Part model, mm, in its own coordinate system. A direction names the side the tool comes from. Round coordinates to 2 decimals unless told otherwise and drop trailing zeros. Write each loop counter-clockwise with the first axis right and the second up, starting at its lowest first coordinate (ties: lowest second). Pieces come first, ordered by that corner, then holes. Notation, with made-up numbers: (-33, 46.25) -> (21, 46.25) arc R22 cw to (21, 73.25) -> close; hole circle Ø2 at (-12.5, -19.5). An arc over 180 degrees is marked (long way). Return JSON: item names as keys, results as strings. Group by question number.
(1) Drop flat-ended pins along their axis: pin 1 Ø1.6 at (y, z) = (-2, 3) entering from -X; pin 2 Ø2.5 at (x, y) = (1.5, -2) entering from +Z; pin 3 Ø1.3 at (x, z) = (0.5, 4.5) entering from +Y. Give the stop position or say it passes through.
(2) Saw through at A-A (z = -21). List the corners of the cut face in (x, y).
(3) Drill centre lines: L1, parallel to X at y = -6.25, z = 1.5; L2, parallel to X at y = -5.25, z = -23; L3, parallel to Y at x = -1.35, z = -6.35 (3 decimals). Where is each one in solid material? Low to high. Write a range as from..to.
(4) Mould opens along X. For faces 4 (the flat face through (-4.324, -2.161, -4.626)), 5 (the cylindrical face through (-8.45, -6.13, 2.94)), 6 (the cylindrical face through (3.684, -3.131, -25.099)) say: +X half, -X half, draft (parallel to the pull), parting line (faces both ways), or undercut.
(5) Tool access for faces 1 (the flat face through (-14, -2, 3)), 2 (the flat face through (-3, -6.35, -13)), 3 (the flat face through (7.8, -13.4, 4.19)): list every direction of +Z, -Z, +X, -X, +Y, -Y with a clear straight run to the whole face (end or side of a thin tool).
(6) Saw through at C-C (z = -6.35). List the corners of the cut face in (x, y) (3 decimals), plus the area to 3 significant figures.
(7) Saw through at B-B (y = -8.25). List the corners of the cut face in (x, z) (3 decimals), plus the area to 3 significant figures.
(8) Saw through at D-D (x = -12.5). List the corners of the cut face in (y, z).
from build123d import *

# Parameters (mm, degrees)
SKETCH1_R                     = 19.05
SKETCH1_R_2                   = 0.5
BOSS_EXTRUDE1_DEPTH           = 6.35
M3_CLEARANCE_HOLE1_D          = 3.2
M3_CLEARANCE_HOLE1_DEPTH      = 29.72
M3_CLEARANCE_HOLE1_TIP        = 0.96137699
SKETCH4_W                     = 37.608509676
SKETCH4_H                     = 0.25
CUT_EXTRUDE1_DEPTH            = 28.679008291
CBORE_FOR_M2_SHCS1_AT_2_COUNT = 2
CBORE_FOR_M2_SHCS1_AT_2_PITCH = 19.05
CUT_EXTRUDE2_DEPTH            = 10
FILLET1_R                     = 2.38125
SKETCH12_W                    = 55.779861043
SKETCH12_H                    = 27.835929003
CUT_EXTRUDE3_DEPTH            = 28.679008452
SKETCH13_W                    = 3
SKETCH13_H                    = 3
BOSS_EXTRUDE2_DEPTH           = 2.5
FILLET2_R                     = 0.5
SKETCH14_W                    = 1.5875
SKETCH14_H                    = 1.4625
CUT_EXTRUDE4_DEPTH            = 28.481584743
SKETCH15_W                    = 3.175
SKETCH15_H                    = 6.35
SKETCH15_W_2                  = 4.7625
BOSS_EXTRUDE3_DEPTH           = 25.4
M2_CLEARANCE_HOLE1_D          = 2.2
M2_CLEARANCE_HOLE1_DEPTH      = 28.35
M2_CLEARANCE_HOLE1_TIP        = 0.660946681
CUT_EXTRUDE5_DEPTH            = 2.5
FILLET3_R                     = 1
FILLET4_R                     = 1


with BuildPart() as part:
    # Sketch1 → Boss-Extrude1 (new body)
    with BuildSketch(Plane.XY):
        Circle(SKETCH1_R)
        with Locations((-12.7, 0)):
            Circle(SKETCH1_R_2, mode=Mode.SUBTRACT)
        with Locations((12.7, 0)):
            Circle(SKETCH1_R_2, mode=Mode.SUBTRACT)
        Circle(SKETCH1_R_2, mode=Mode.SUBTRACT)
    extrude(amount=BOSS_EXTRUDE1_DEPTH)

    # M3 Clearance Hole1
    with Locations(Plane(origin=(-15.665967818, 20.219646462, 6.35), x_dir=(1, 0, 0), z_dir=(0, 0, 1))):
        with Locations((15.665967818, -5.554949625), (2.965967818, -27.551994881), (28.365967818, -27.551994881)):
            Hole(M3_CLEARANCE_HOLE1_D / 2, depth=M3_CLEARANCE_HOLE1_DEPTH)
            with Locations((0, 0, -(M3_CLEARANCE_HOLE1_DEPTH + M3_CLEARANCE_HOLE1_TIP / 2))):  # 118° drill point
                Cone(0, M3_CLEARANCE_HOLE1_D / 2, M3_CLEARANCE_HOLE1_TIP, mode=Mode.SUBTRACT)

    # Sketch4 → Cut-Extrude1 (cut, through all)
    with BuildSketch(Plane(origin=(0, 0, 0), x_dir=(-1, 0, 0), z_dir=(0, 0, -1))):
        with Locations((0, -3.175)):
            Rectangle(SKETCH4_W, SKETCH4_H)
    extrude(amount=-CUT_EXTRUDE1_DEPTH, mode=Mode.SUBTRACT)


with BuildPart() as cut_extrude1_piece_1:
    # of the separate pieces the step leaves, piece 1, a body of its own (cut_extrude1_pieces)
    add(part.part.solids().sort_by_distance((18.804254838, -3.05, 0))[0])


with BuildPart() as cut_extrude1_piece_2:
    # of the separate pieces the step leaves, piece 2, a body of its own (cut_extrude1_pieces)
    add(part.part.solids().sort_by_distance((-18.761996162, -3.3, 0))[0])


with BuildPart() as cbore_for_m2_shcs1_tool:
    # Sketch9 → CBORE for M2 SHCS1 (revolve)
    with BuildSketch(Plane(origin=(-9.525, 19.05, 3.175), x_dir=(0, 0, 1), z_dir=(1, 0, 0))):
        Polygon((0, 0), (0, 38.1), (1.1, 38.1), (1.1, 2), (2.2, 2), (2.2, 0), align=None)
    cbore_for_m2_shcs1 = revolve(axis=Axis((-9.525, 25.4, 3.175), (0, -1, 0)))


with BuildPart() as cut_extrude1_piece_1_1:
    add(cut_extrude1_piece_1.part)

    # CBORE for M2 SHCS1: cut by cbore_for_m2_shcs1_tool
    add(cbore_for_m2_shcs1_tool.part, mode=Mode.SUBTRACT)


with BuildPart() as cut_extrude1_piece_2_1:
    add(cut_extrude1_piece_2.part)

    # CBORE for M2 SHCS1: cut by cbore_for_m2_shcs1_tool
    add(cbore_for_m2_shcs1_tool.part, mode=Mode.SUBTRACT)


with BuildPart() as cbore_for_m2_shcs1_at_2_tool:
    # CBORE for M2 SHCS1 at 2: CBORE for M2 SHCS1 ×2
    with Locations(*[(i * CBORE_FOR_M2_SHCS1_AT_2_PITCH, 0, 0) for i in range(1, CBORE_FOR_M2_SHCS1_AT_2_COUNT)]):
        add(cbore_for_m2_shcs1)


with BuildPart() as cut_extrude1_piece_1_2:
    add(cut_extrude1_piece_1_1.part)

    # CBORE for M2 SHCS1 at 2: cut by cbore_for_m2_shcs1_at_2_tool
    add(cbore_for_m2_shcs1_at_2_tool.part, mode=Mode.SUBTRACT)

    # Fillet1
    fillet1_edges = [cut_extrude1_piece_1_2.edges().sort_by_distance(p)[0] for p in [
        (-0.5, 0, 0),
        (-13.2, 0, 0),
        (12.2, 0, 0),
        (-13.2, 0, 6.35),
        (12.2, 0, 6.35),
        (-0.5, 0, 6.35),
    ]]
    fillet(fillet1_edges, radius=FILLET1_R)

    # Sketch12 → Cut-Extrude3 (cut, through all)
    with BuildSketch(Plane.XY):
        with Locations((0.042756797, 10.867964502)):
            Rectangle(SKETCH12_W, SKETCH12_H)
    extrude(amount=CUT_EXTRUDE3_DEPTH, mode=Mode.SUBTRACT)


with BuildPart() as cut_extrude1_piece_2_2:
    add(cut_extrude1_piece_2_1.part)

    # CBORE for M2 SHCS1 at 2: cut by cbore_for_m2_shcs1_at_2_tool
    add(cbore_for_m2_shcs1_at_2_tool.part, mode=Mode.SUBTRACT)

    # Sketch11 → Cut-Extrude2 (cut)
    with BuildSketch(Plane.XZ.offset(19.05)):
        Polygon((-10.679700538, 5.175), (-11.834401077, 3.175), (-10.679700538, 1.175), (-8.370299462, 1.175), (-7.215598923, 3.175), (-8.370299462, 5.175), align=None)
        Polygon((8.370299462, 5.175), (7.215598923, 3.175), (8.370299462, 1.175), (10.679700538, 1.175), (11.834401077, 3.175), (10.679700538, 5.175), align=None)
    extrude(amount=-CUT_EXTRUDE2_DEPTH, mode=Mode.SUBTRACT)

    # Sketch13 → Boss-Extrude2 (add)
    with BuildSketch(Plane(origin=(0, -3.3, 0), x_dir=(1, 0, 0), z_dir=(0, 1, 0))):
        with Locations((-15.5, -3.175)):
            Rectangle(SKETCH13_W, SKETCH13_H)
        with Locations((15.5, -3.175)):
            Rectangle(SKETCH13_W, SKETCH13_H)
    extrude(amount=BOSS_EXTRUDE2_DEPTH)

    # Fillet2
    fillet2_edges = [cut_extrude1_piece_2_2.edges().sort_by_distance(p)[0] for p in [
        (17, -3.3, 3.175),
        (17, -2.05, 4.675),
        (15.5, -3.3, 1.675),
        (17, -2.05, 1.675),
        (14, -3.3, 3.175),
        (14, -2.05, 1.675),
        (15.5, -3.3, 4.675),
        (14, -2.05, 4.675),
        (17, -0.8, 3.175),
        (15.5, -0.8, 1.675),
        (14, -0.8, 3.175),
        (15.5, -0.8, 4.675),
        (-15.5, -3.3, 1.675),
        (-14, -2.05, 1.675),
        (-17, -3.3, 3.175),
        (-17, -2.05, 1.675),
        (-15.5, -3.3, 4.675),
        (-17, -2.05, 4.675),
        (-14, -3.3, 3.175),
        (-14, -2.05, 4.675),
        (-15.5, -0.8, 1.675),
        (-17, -0.8, 3.175),
        (-15.5, -0.8, 4.675),
        (-14, -0.8, 3.175),
    ]]
    fillet(fillet2_edges, radius=FILLET2_R)

    # Sketch14 → Cut-Extrude4 (cut, through all)
    with BuildSketch(Plane(origin=(0, 0, 0), x_dir=(-1, 0, 0), z_dir=(0, 0, -1))):
        with Locations((0, -4.03125)):
            Rectangle(SKETCH14_W, SKETCH14_H)
    extrude(amount=-CUT_EXTRUDE4_DEPTH, mode=Mode.SUBTRACT)

    # Sketch15 → Boss-Extrude3 (add)
    with BuildSketch(Plane(origin=(0, 0, 0), x_dir=(-1, 0, 0), z_dir=(0, 0, -1))):
        with Locations((-2.38125, -3.175)):
            Rectangle(SKETCH15_W, SKETCH15_H)
        with Locations((3.175, -3.175)):
            Rectangle(SKETCH15_W_2, SKETCH15_H)
    extrude(amount=BOSS_EXTRUDE3_DEPTH)

    # M2 Clearance Hole1
    with Locations(Plane.ZY.offset(5.55625)):
        with Locations((-6.35, -3.175)):
            Hole(M2_CLEARANCE_HOLE1_D / 2, depth=M2_CLEARANCE_HOLE1_DEPTH)
            with Locations((0, 0, -(M2_CLEARANCE_HOLE1_DEPTH + M2_CLEARANCE_HOLE1_TIP / 2))):  # 118° drill point
                Cone(0, M2_CLEARANCE_HOLE1_D / 2, M2_CLEARANCE_HOLE1_TIP, mode=Mode.SUBTRACT)

    # Sketch18 → Cut-Extrude5 (cut)
    with BuildSketch(Plane.ZY.offset(5.55625)):
        Polygon((-7.504700538, -1.175), (-5.195299462, -1.175), (-4.040598923, -3.175), (-5.195299462, -5.175), (-7.504700538, -5.175), (-8.659401077, -3.175), align=None)
    extrude(amount=-CUT_EXTRUDE5_DEPTH, mode=Mode.SUBTRACT)

    # Fillet3
    fillet3_edges = [cut_extrude1_piece_2_2.edges().sort_by_distance(p)[0] for p in [
        (3.96875, -4.825, 0),
        (2.38125, -6.35, 0),
        (0.79375, -3.175, -25.4),
        (2.38125, 0, -25.4),
        (3.96875, -3.175, -25.4),
        (2.38125, -6.35, -25.4),
        (-3.175, -6.35, 0),
        (-5.55625, -4.825, 0),
        (-0.79375, -3.175, -25.4),
        (-3.175, -6.35, -25.4),
        (-5.55625, -3.175, -25.4),
        (-3.175, 0, -25.4),
    ]]
    fillet(fillet3_edges, radius=FILLET3_R)

    # Fillet4
    fillet4_edges = [cut_extrude1_piece_2_2.edges().sort_by_distance(p)[0] for p in [
        (2.38125, 0, 0),
        (-3.175, 0, 0),
    ]]
    fillet(fillet4_edges, radius=FILLET4_R)


solid = cut_extrude1_piece_2_2.part
Computed values:
{
 "1": {"pin 1": "x = -17", "pin 2": "z = 0", "pin 3": "y = -3.3"},
 "2": {"outline": "(-5.56, -6.35) -> (-0.79, -6.35) -> (-0.79, 0) -> (-5.56, 0) -> close; (0.79, -6.35) -> (3.97, -6.35) -> (3.97, 0) -> (0.79, 0) -> close"},
 "3": {"L1": "-18..-13.88, -11.52..11.52, 13.88..18", "L2": "-5.56..-0.79, 0.79..3.97", "L3": "-6.35..-4.275, -2.075..0"},
 "4": {"face 4": "draft", "face 5": "undercut", "face 6": "+X half"},
 "5": {"face 1": "+Z, -Z, +Y", "face 2": "-Z, +X, -X, -Y", "face 3": "-Y"},
 "6": {"outline": "(-5.556, -6.35) -> (-0.794, -6.35) -> (-0.794, -4.275) -> (-3.056, -4.275) -> (-3.056, -5.175) -> (-5.556, -5.175) -> close; (-5.556, -1.175) -> (-3.056, -1.175) -> (-3.056, -2.075) -> (-0.794, -2.075) -> (-0.794, 0) -> (-5.556, 0) -> close; (0.794, -6.35) -> (3.969, -6.35) -> (3.969, -4.275) -> (0.794, -4.275) -> close; (0.794, -2.075) -> (3.969, -2.075) -> (3.969, 0) -> (0.794, 0) -> close", "area": "28.4 mm2"},
 "7": {"outline": "(-17.171, 0) -> (-14.011, 0) -> (-14.011, 6.35) -> (-17.171, 6.35) -> close; (-11.389, 0) -> (11.389, 0) -> (11.389, 6.35) -> (-11.389, 6.35) -> close; (14.011, 0) -> (17.171, 0) -> (17.171, 6.35) -> (14.011, 6.35) -> close; hole circle Ø2.2 at (-9.525, 3.175); hole circle Ø2.2 at (9.525, 3.175)", "area": "177 mm2"},
 "8": {"outline": "(-14.38, 0) -> (-8.92, 0) -> (-8.92, 6.35) -> (-14.38, 6.35) -> close; (-5.74, 0) -> (-3.3, 0) -> (-3.3, 6.35) -> (-5.74, 6.35) -> close"}
}
